from build123d import *

# Parameters (mm, degrees)
F1_DEPTH = 3


with BuildPart() as f1:
    # F0 (on Front) → F1 (new body)
    with BuildSketch(Plane.XZ):
        with BuildLine():
            Line((-6, -17.5), (6, -17.5))
            Line((6, -17.5), (6, 17.5))
            Line((6, 17.5), (9, 17.5))
            ThreePointArc((9, 17.5), (7.535534, 21.035534), (4, 22.5))
            Line((4, 22.5), (-4, 22.5))
            ThreePointArc((-4, 22.5), (-7.535534, 21.035534), (-9, 17.5))
            Line((-9, 17.5), (-6, 17.5))
            Line((-6, 17.5), (-6, -11.5))
            Line((-6, -11.5), (0, -11.5))
            Line((0, -11.5), (0, -14.5))
            Line((0, -14.5), (-6, -14.5))
            Line((-6, -14.5), (-6, -17.5))
        make_face()
    extrude(amount=F1_DEPTH)


solid = f1.part
Read the model definition and answer for the solid it produces. Units are mm, in the model's axes. A direction names the side the tool comes from. Round coordinates to 2 decimals unless told otherwise and drop trailing zeros. Loops run counter-clockwise (first coordinate to the right, second up) from the corner with the lowest first, then second, coordinate; pieces in that order, holes last. Notation, with made-up numbers: (70.25, 87.5) - (79.25, 87.5) arc R27 ccw to (79.25, 121.5) - close; hole circle Ø8 at (-10, -15.5). An arc over 180 degrees is marked (long way). One line per question, with ' | ' between items. Start each with the question number.
Q1. Find the intervals of material crossed by L1, parallel to Z at x = -2.75, y = -1.25; L2, parallel to X at y = -0.35, z = -1; L3, parallel to X at y = -0.3, z = -13.5, in increasing order.
Q2. Section A-A on x = -3.5 is taken. Give the vertices of the cut face in (y, z).
Q3. For faces 4 (the flat face through (-8, -1, 17.5)), 5 (the flat face through (6, -1, 0)), 6 (the flat face through (0, -1, -13)), determine the directions among +Z, -Z, +X, -X, +Y, -Y from which every point of the face is accessible in a straight line to the end or side of a thin tool.
Q4. Section C-C on z = 13 is taken. Give the vertices of the cut face in (x, y).
Q5. Section D-D on x = 6.5 is taken. Give the vertices of the cut face in (y, z), plus the area to 3 significant figures.
Q6. Flat-ended cylindrical pins translate along their axes: pin 1 (1.5 mm diameter, centred on y = -1, z = 7.5, fed in from -X); pin 2 (0.9 mm diameter, centred on x = 7, y = -1.5, fed in from -Z); pin 3 (0.9 mm diameter, centred on y = -1.5, z = 5.5, fed in from +X). Find the tip coordinate at first contact, or state that the pin passes through.
Q7. For a pull along Z with two mould halves and no side action, classify faces 1 (the cylindrical face through (7.57, -1.48, 21)), 2 (the flat face through (-3, -1, -14.5)), 3 (the flat face through (-6, -1, -16)) as +Z half, -Z half, draft (parallel to the pull), parting line (faces both ways), or undercut.
Q8. Section B-B on y = -1.8 is taken. Give the vertices of the cut face in (x, z), plus the area to 3 significant figures.
Established:
1) L1: -17.5 to -14.5, -11.5 to 22.5 | L2: -6 to 6 | L3: 0 to 6
2) outline: (-3, -17.5) - (0, -17.5) - (0, -14.5) - (-3, -14.5) - close; (-3, -11.5) - (0, -11.5) - (0, 22.5) - (-3, 22.5) - close
3) face 4: -Z, -X, +Y, -Y | face 5: -Z, +X, +Y, -Y | face 6: -X, +Y, -Y
4) outline: (-6, -3) - (6, -3) - (6, 0) - (-6, 0) - close
5) outline: (-3, 17.5) - (0, 17.5) - (0, 21.83) - (-3, 21.83) - close | area: 13.0 mm²
6) pin 1: x = -6 | pin 2: z = 17.5 | pin 3: x = 6
7) face 1: +Z half | face 2: undercut | face 3: draft
8) outline: (-9, 17.5) - (-6, 17.5) - (-6, -11.5) - (0, -11.5) - (0, -14.5) - (-6, -14.5) - (-6, -17.5) - (6, -17.5) - (6, 17.5) - (9, 17.5) arc R5 ccw to (4, 22.5) - (-4, 22.5) arc R5 ccw to start | area: 481 mm²
